The listing builds one solid part. Answer for the finished solid, in the listing's coordinates (mm). Round coordinates to 2 decimals unless told otherwise and drop trailing zeros. Write each loop counter-clockwise with the first axis right and the second up, starting at its lowest first coordinate (ties: lowest second). Pieces come first, ordered by that corner, then holes. Notation, with made-up numbers: (-12.5, 68.25) - (14.5, 68.25) arc R16 cw to (14.5, 99.25) - close; hole circle Ø8 at (65.25, 29.5). An arc over 180 degrees is marked (long way). Return JSON: item names as keys, results as strings. Group by question number.
(1) Each of these flat-tipped pins is pushed along its axis until it touches: pin 1 (1 mm diameter, centred on x = -2, z = 334.5, fed in from +Y); pin 2 (1 mm diameter, centred on y = 5.5, z = 221, fed in from +X); pin 3 (1.5 mm diameter, centred on x = 5, z = 358, fed in from +Y); pin 4 (5.5 mm diameter, centred on y = -1, z = 9, fed in from -X). Where does it stop, or does it pass through?
(2) Find the intervals of material crossed by line 1 along Z through (x, y) = (-8.5, 0); line 2 along Z through (x, y) = (-8.75, -1); line 3 along Y through (x, z) = (0.5, 427.5), in increasing order. Write a range as [from, to].
(3) Section A-A, the plane y = 0 is taken. Write down the section's boundary in (x, z).
```python
from build123d import *

# Parameters (mm, degrees)
F0_R     = 12.7
F1_DEPTH = 499.999
F2_R     = 6.35
F3_DEPTH = 76.2
F4_R     = 6.35
F5_DEPTH = 76.2


with BuildPart() as f1:
    # F0 (on Top) → F1 (new body)
    with BuildSketch(Plane.XY):
        Circle(F0_R)
    extrude(amount=F1_DEPTH)

    # F2 (on Right) → F3 (cut)
    with BuildSketch(Plane.YZ):
        with Locations((0, 11.162438)):
            Circle(F2_R)
    extrude(amount=F3_DEPTH, mode=Mode.SUBTRACT)

    # F4 (on Right) → F5 (cut)
    with BuildSketch(Plane.YZ):
        with Locations((0, 10.668855)):
            Circle(F4_R)
    extrude(amount=-F5_DEPTH, mode=Mode.SUBTRACT)


solid = f1.part
```
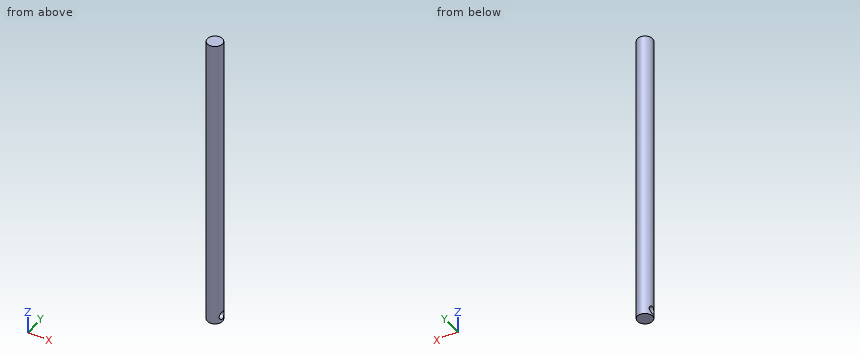
Working result:
{
 "1": {"pin 1": "stops at y = 12.61", "pin 2": "stops at x = 11.67", "pin 3": "stops at y = 11.97", "pin 4": "passes through"},
 "2": {"line 1": "z = [0, 4.32], [17.02, 500]", "line 2": "z = [0, 4.4], [16.94, 500]", "line 3": "y = [-12.69, 12.69]"},
 "3": {"outline": "(-12.7, 0) - (12.7, 0) - (12.7, 4.81) - (0, 4.81) - (0, 4.32) - (-12.7, 4.32) - close; (-12.7, 17.02) - (0, 17.02) - (0, 17.51) - (12.7, 17.51) - (12.7, 500) - (-12.7, 500) - close"}
}
